Can you work these out from the model? Positions are in its coordinate system, mm. Face numbers are marked on the shaded views. A direction names the side the tool comes from. Coordinates: 2 decimals unless noted, no trailing zeros. Write each loop counter-clockwise with the first axis right and the second up, starting at its lowest first coordinate (ties: lowest second). Pieces come first, ordered by that corner, then holes. Notation, with made-up numbers: (-0.5, 24) -> (42.5, 24) arc R26 ccw to (42.5, 50) -> close; hole circle Ø2 at (69.5, 36). An arc over 180 degrees is marked (long way). Use one line per item in the form item = value.
```python
from build123d import *

# Parameters (mm, degrees)
SKETCH1_R               = 25
BOSS_EXTRUDE1_DEPTH     = 5
CUT_EXTRUDE1_START      = 5
CUT_EXTRUDE1_DEPTH      = 2.6
SKETCH1_5_R             = 1.05
CUT_EXTRUDE2_DEPTH      = 6
CUT_EXTRUDE4_DEPTH      = 1.6
CUT_EXTRUDE5_DEPTH      = 1.6
SKETCH5_W               = 7
SKETCH5_H               = 25
CUT_EXTRUDE6_DEPTH      = 4.2
SKETCH6_W               = 10.9
SKETCH6_H               = 5
CUT_EXTRUDE7_DEPTH      = 5.2
SKETCH7_W               = 1
SKETCH7_H               = 1
SKETCH8_R               = 1.05
CUT_EXTRUDE8_DEPTH      = 26
CUT_EXTRUDE8_DEPTH_BACK = 26


with BuildPart() as part:
    # Sketch1 → Boss-Extrude1 (new body)
    with BuildSketch(Plane(origin=(0, 0, 0), x_dir=(1, 0, 0), z_dir=(0, 1, 0))):
        Circle(SKETCH1_R)
    extrude(amount=BOSS_EXTRUDE1_DEPTH)

    # Sketch1<4> → Cut-Extrude1 (cut)
    with BuildSketch(Plane(origin=(0, 0, 0), x_dir=(1, 0, 0), z_dir=(0, 1, 0)).offset(CUT_EXTRUDE1_START)):
        with BuildLine():
            ThreePointArc((-7.646663173, 15.290666359), (-14.941166286, 14.941166286), (-15.290666359, 7.646663173))
            ThreePointArc((-15.290666359, 7.646663173), (-14.860391858, 6.700345618), (-14.963208205, 5.665898006))
            ThreePointArc((-14.963208205, 5.665898006), (-16, 0), (-14.963208205, -5.665898006))
            ThreePointArc((-14.963208205, -5.665898006), (-14.860391858, -6.700345618), (-15.290666359, -7.646663173))
            ThreePointArc((-15.290666359, -7.646663173), (-14.941166286, -14.941166286), (-7.646663173, -15.290666359))
            ThreePointArc((-7.646663173, -15.290666359), (-6.700345618, -14.860391858), (-5.665898006, -14.963208205))
            ThreePointArc((-5.665898006, -14.963208205), (0, -16), (5.665898006, -14.963208205))
            ThreePointArc((5.665898006, -14.963208205), (6.700345618, -14.860391858), (7.646663173, -15.290666359))
            ThreePointArc((7.646663173, -15.290666359), (14.941166286, -14.941166286), (15.290666359, -7.646663173))
            ThreePointArc((15.290666359, -7.646663173), (14.860391858, -6.700345618), (14.963208205, -5.665898006))
            ThreePointArc((14.963208205, -5.665898006), (16, 0), (14.963208205, 5.665898006))
            ThreePointArc((14.963208205, 5.665898006), (14.860391858, 6.700345618), (15.290666359, 7.646663173))
            ThreePointArc((15.290666359, 7.646663173), (14.941166286, 14.941166286), (7.646663173, 15.290666359))
            ThreePointArc((7.646663173, 15.290666359), (6.700345618, 14.860391858), (5.665898006, 14.963208205))
            ThreePointArc((5.665898006, 14.963208205), (0, 16), (-5.665898006, 14.963208205))
            ThreePointArc((-5.665898006, 14.963208205), (-6.700345618, 14.860391858), (-7.646663173, 15.290666359))
        make_face()
    extrude(amount=-CUT_EXTRUDE1_DEPTH, mode=Mode.SUBTRACT)

    # Sketch1<5> → Cut-Extrude2 (cut, through all)
    with BuildSketch(Plane(origin=(0, 0, 0), x_dir=(1, 0, 0), z_dir=(0, 1, 0))):
        with Locations((12.105668094, 12.105668094)):
            Circle(SKETCH1_5_R)
        with Locations((12.105668094, -12.105668094)):
            Circle(SKETCH1_5_R)
        with Locations((-12.105668094, -12.105668094)):
            Circle(SKETCH1_5_R)
        with Locations((-12.105668094, 12.105668094)):
            Circle(SKETCH1_5_R)
    extrude(amount=CUT_EXTRUDE2_DEPTH, mode=Mode.SUBTRACT)

    # Sketch3 → Cut-Extrude4 (cut)
    with BuildSketch(Plane(origin=(0, 2.4, 0), x_dir=(1, 0, 0), z_dir=(0, 1, 0))):
        with BuildLine():
            Line((-14.250424192, -7.548306686), (-13.078556304, -6.927580025))
            ThreePointArc((-13.078556304, -6.927580025), (-10.465180362, -10.465180362), (-6.927580025, -13.078556304))
            Line((-6.927580025, -13.078556304), (-7.548306686, -14.250424192))
            Line((-7.548306686, -14.250424192), (-5.665898006, -14.963208205))
            ThreePointArc((-5.665898006, -14.963208205), (0, -16), (5.665898006, -14.963208205))
            Line((5.665898006, -14.963208205), (7.548306686, -14.250424192))
            Line((7.548306686, -14.250424192), (6.927580025, -13.078556304))
            ThreePointArc((6.927580025, -13.078556304), (10.465180362, -10.465180362), (13.078556304, -6.927580025))
            Line((13.078556304, -6.927580025), (14.250424192, -7.548306686))
            Line((14.250424192, -7.548306686), (14.963208205, -5.665898006))
            ThreePointArc((14.963208205, -5.665898006), (16, 0), (14.963208205, 5.665898006))
            Line((14.963208205, 5.665898006), (14.250424192, 7.548306686))
            Line((14.250424192, 7.548306686), (13.078556304, 6.927580025))
            ThreePointArc((13.078556304, 6.927580025), (10.465180362, 10.465180362), (6.927580025, 13.078556304))
            Line((6.927580025, 13.078556304), (7.548306686, 14.250424192))
            Line((7.548306686, 14.250424192), (5.665898006, 14.963208205))
            ThreePointArc((5.665898006, 14.963208205), (0, 16), (-5.665898006, 14.963208205))
            Line((-5.665898006, 14.963208205), (-7.548306686, 14.250424192))
            Line((-7.548306686, 14.250424192), (-6.927580025, 13.078556304))
            ThreePointArc((-6.927580025, 13.078556304), (-10.465180362, 10.465180362), (-13.078556304, 6.927580025))
            Line((-13.078556304, 6.927580025), (-14.250424192, 7.548306686))
            Line((-14.250424192, 7.548306686), (-14.963208205, 5.665898006))
            ThreePointArc((-14.963208205, 5.665898006), (-16, 0), (-14.963208205, -5.665898006))
            Line((-14.963208205, -5.665898006), (-14.250424192, -7.548306686))
        make_face()
    extrude(amount=-CUT_EXTRUDE4_DEPTH, mode=Mode.SUBTRACT)

    # Sketch4 → Cut-Extrude5 (cut)
    with BuildSketch(Plane.XZ):
        Polygon((-10.391025274, 13.820310914), (-12.733270924, 14.447913744), (-14.447913744, 12.733270924), (-13.820310914, 10.391025274), (-11.478065263, 9.763422443), (-9.763422443, 11.478065263), align=None)
        Polygon((13.820310914, 10.391025274), (14.447913744, 12.733270924), (12.733270924, 14.447913744), (10.391025274, 13.820310914), (9.763422443, 11.478065263), (11.478065263, 9.763422443), align=None)
        Polygon((10.391025274, -13.820310914), (12.733270924, -14.447913744), (14.447913744, -12.733270924), (13.820310914, -10.391025274), (11.478065263, -9.763422443), (9.763422443, -11.478065263), align=None)
        Polygon((-13.820310914, -10.391025274), (-14.447913744, -12.733270924), (-12.733270924, -14.447913744), (-10.391025274, -13.820310914), (-9.763422443, -11.478065263), (-11.478065263, -9.763422443), align=None)
    extrude(amount=-CUT_EXTRUDE5_DEPTH, mode=Mode.SUBTRACT)

    # Sketch5 → Cut-Extrude6 (cut)
    with BuildSketch(Plane(origin=(0, 5, 0), x_dir=(1, 0, 0), z_dir=(0, 1, 0))):
        with Locations((0, -12.5)):
            Rectangle(SKETCH5_W, SKETCH5_H)
    extrude(amount=-CUT_EXTRUDE6_DEPTH, mode=Mode.SUBTRACT)

    # Sketch6 → Cut-Extrude7 (cut, through all)
    with BuildSketch(Plane(origin=(0, 0.8, 0), x_dir=(1, 0, 0), z_dir=(0, 1, 0))):
        with Locations((0, -22.5)):
            Rectangle(SKETCH6_W, SKETCH6_H)
    extrude(amount=CUT_EXTRUDE7_DEPTH, mode=Mode.SUBTRACT)

    # Sketch7 → Cut-Revolve1 (revolve, cut)
    with BuildSketch(Plane.XY):
        Polygon((-25, 1), (-24, 0), (-25, 0), align=None)
        with Locations((-24.5, 4.5)):
            Rectangle(SKETCH7_W, SKETCH7_H)
    revolve(axis=Axis((0, 5.25, 0), (0, -1, 0)), mode=Mode.SUBTRACT)

    # Sketch8 → Cut-Extrude8 (cut, two sides)
    with BuildSketch(Plane(origin=(0, 0, 0), x_dir=(0, 0, -1), z_dir=(1, 0, 0))) as cut_extrude8_sk:
        with Locations((0, 3)):
            Circle(SKETCH8_R)
    extrude(amount=CUT_EXTRUDE8_DEPTH, mode=Mode.SUBTRACT)
    extrude(cut_extrude8_sk.sketch, amount=-CUT_EXTRUDE8_DEPTH_BACK, mode=Mode.SUBTRACT)


solid = part.part
```
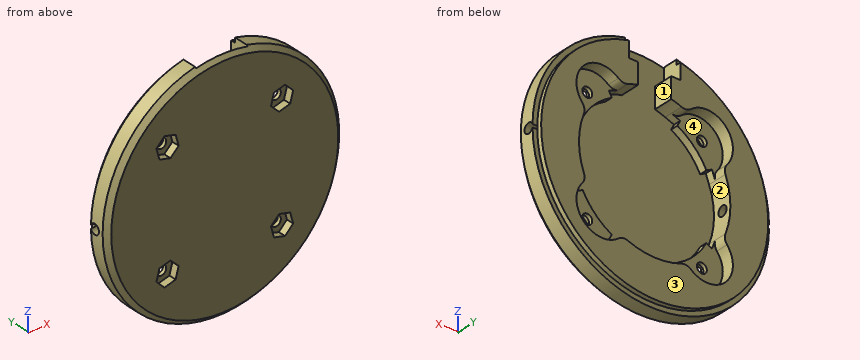
Q1. For the marked faces 3 and 4, which set-ups out of +Z, -Z, +X, -X, +Y, -Y let a thin tool reach every point of the face, with its end or its side?
Return value:
face_3 = +Z, -Z, +X, -X, +Y
face_4 = +Y
Q2. Suppose I cut it at A-A (y = 3). Give the number of separate pieces and of enclosed holes in the cut face, then the cut area to 3 significant figures.
Return value:
separate_pieces = 3
enclosed_holes = 0
area = 852 mm2
Q3. Suppose I cut it at B-B (x = 0). Write out the boundary of the cut face in (y, z), then the cut area to 3 significant figures.
Return value:
outline = (0, -24) -> (1, -25) -> (4, -25) -> (4, -24) -> (5, -24) -> (5, -16) -> (0.8, -16) -> (0.8, 24.8) -> (0, 24) -> close
area = 75.8 mm2
Q4. Will these pins go through, and if not, where does the flat tip stop? pin 1 (2 mm diameter, centred on x = 13.5, z = 14, fed in from -Y); pin 2 (2 mm diameter, centred on x = -4.5, y = 3.5, fed in from +Z); pin 3 (1 mm diameter, centred on y = 0.5, z = -16, fed in from +X); pin 4 (2 mm diameter, centred on y = 3, z = 4, fed in from -X).
Return value:
pin_1 = 0
pin_2 = 24.4
pin_3 = 19.33
pin_4 = -24.82
Q5. If I drill on line 1 (X direction, y = 0.6, z = 13); line 2 (Y direction, x = -22.5, z = 0); line 3 (X direction, y = 1.25, z = -11.5), over which ranges is the centre line in solid material (lowest first)? Write a range as from..to.
Return value:
line_1 = -20.88..-14.18, -10.17..10.17, 14.18..20.88
line_2 = 0..1.95, 4.05..5
line_3 = -22.2..-14.12, -9.77..-9.32, 9.32..9.77, 14.12..22.2
Q6. Thinking about a two-plate mould opening in Z: for the marked faces 1 and 2, which applies, released by +Z, released by -Z, zero draft, split by the parting line, or undercut?
Return value:
face_1 = zero draft
face_2 = undercut
